Could you check a few things on this model? Use its own coordinates, in mm. A direction names the side the tool comes from. Coordinates: 2 decimals unless noted, no trailing zeros. Order: outer loops, then holes, each group sorted by start corner. A loop starts at its lowest first (then second) coordinate and runs counter-clockwise, first axis right, second up. Notation, with made-up numbers: (10.5, -18.5) - (28.5, -18.5) arc R24 cw to (28.5, 2.5) - close; hole circle Ø6 at (23, 18.25). An arc over 180 degrees is marked (long way). One line per item, written item: value. Start each with the question number.
from build123d import *

# Parameters (mm, degrees)
SALIENTE_EXTRUIR1_DEPTH = 3
CROQUIS2_R              = 1.5
CORTAR_EXTRUIR2_DEPTH   = 4
SALIENTE_EXTRUIR2_DEPTH = 10


with BuildPart() as part:
    # Croquis1 → Saliente-Extruir1 (new body)
    with BuildSketch(Plane(origin=(0, 0, 0), x_dir=(1, 0, 0), z_dir=(0, 1, 0))):
        Polygon((-16.25, 29), (-16.25, -6), (39.25, -6), (39.25, -29), (-39.25, -29), (-39.25, 29), align=None)
    extrude(amount=SALIENTE_EXTRUIR1_DEPTH)

    # Croquis2 → Cortar-Extruir2 (cut, through all)
    with BuildSketch(Plane(origin=(0, 3, 0), x_dir=(1, 0, 0), z_dir=(0, 1, 0))):
        with Locations((31.75, -20.05)):
            Circle(CROQUIS2_R)
        with Locations((16.75, -20.05)):
            Circle(CROQUIS2_R)
        with Locations((-30.3, 22.75)):
            Circle(CROQUIS2_R)
        with Locations((-30.3, 7.75)):
            Circle(CROQUIS2_R)
    extrude(amount=-CORTAR_EXTRUIR2_DEPTH, mode=Mode.SUBTRACT)

    # Croquis3 → Saliente-Extruir2 (add)
    with BuildSketch(Plane(origin=(0, 3, 0), x_dir=(1, 0, 0), z_dir=(0, 1, 0))):
        Polygon((-16.25, 29), (-16.25, -6), (39.25, -6), (39.25, -4.5), (-14.75, -4.5), (-14.75, 29), align=None)
    extrude(amount=-SALIENTE_EXTRUIR2_DEPTH)


solid = part.part
Q1. I want a section at D-D on y = -3.25. Please give me the cut outline in (x, z), then the cut area to 4 significant figures.
Q2. Which directions (+Z, -Z, +X, -X, +Y, -Y) give clear straight access to the entire face, cutting with the end or side of a thin tool? Please do faces 1 (the flat face through (-16.25, -3, -12)), 2 (the flat face through (-14.75, -2, -12)), 3 (the flat face through (11, -3, 6)).
Q3. I want a section at B-B on z = 20.05. Please give me the cut outline in (x, y), then the cut area to 4 significant figures.
Q4. If I drill on L1, parallel to X at y = 1.85, z = 20.05; L2, parallel to Z at x = -30.3, y = 2.25; L3, parallel to Z at x = 16.75, y = 1.8, over which ranges is the centre line in solid material (lowest first)?
Q5. We'd pull the mould along X, two halves only. Please class faces 4 (the flat face through (1, 1, 29)), 5 (the cylindrical face through (15.64, 1.52, 19.04)), 6 (the flat face through (39.25, 0.2, 13.9)): +X half, -X half, draft (parallel to the pull), parting line (faces both ways), or undercut.
Q6. I want a section at C-C on y = 1.75. Please give me the cut outline in (x, z).
Q7. I want a section at A-A on x = -30.3. Please give me the cut outline in (y, z).
Q8. I'm going to push flat-ended pins straight in: pin 1 (5 mm diameter, centred on y = -1.5, z = -21.5, fed in from +X); pin 2 (5 mm diameter, centred on x = 23.5, y = -0.5, fed in from -Z); pin 3 (2 mm diameter, centred on x = 18, y = -3, fed in from +Z). Where does each tip first touch, or does it pass through?
Values follow:
1. outline: (-16.25, -29) - (-14.75, -29) - (-14.75, 4.5) - (39.25, 4.5) - (39.25, 6) - (-16.25, 6) - close
1. area: 133.5 mm^2
2. face 1: +Z, -Z, -X, -Y
2. face 2: -Z, +X, +Y, -Y
2. face 3: +Z, +X, -X, -Y
3. outline: (-39.25, 0) - (15.25, 0) - (15.25, 3) - (-39.25, 3) - close; (18.25, 0) - (30.25, 0) - (30.25, 3) - (18.25, 3) - close; (33.25, 0) - (39.25, 0) - (39.25, 3) - (33.25, 3) - close
3. area: 217.5 mm^2
4. L1: x = -39.25 to 15.25, 18.25 to 30.25, 33.25 to 39.25
4. L2: z = -29 to -24.25, -21.25 to -9.25, -6.25 to 29
4. L3: z = 4.5 to 18.55, 21.55 to 29
5. face 4: draft
5. face 5: undercut
5. face 6: +X half
6. outline: (-39.25, -29) - (-14.75, -29) - (-14.75, 4.5) - (39.25, 4.5) - (39.25, 29) - (-39.25, 29) - close; hole circle Ø3 at (-30.3, -22.75); hole circle Ø3 at (-30.3, -7.75); hole circle Ø3 at (16.75, 20.05); hole circle Ø3 at (31.75, 20.05)
7. outline: (0, -29) - (3, -29) - (3, -24.25) - (0, -24.25) - close; (0, -21.25) - (3, -21.25) - (3, -9.25) - (0, -9.25) - close; (0, -6.25) - (3, -6.25) - (3, 29) - (0, 29) - close
8. pin 1: stops at x = -14.75
8. pin 2: stops at z = 4.5
8. pin 3: stops at z = 6
